```python
from build123d import *

# Parameters (mm, degrees)
CROQUIS1_R              = 2.55
CROQUIS1_R_2            = 1.55
SALIENTE_EXTRUIR1_DEPTH = 3
REDONDEO2_R             = 2
CORTAR_EXTRUIR1_DEPTH   = 3


with BuildPart() as part:
    # Croquis1 → Saliente-Extruir1 (new body)
    with BuildSketch(Plane(origin=(0, 0, 0), x_dir=(1, 0, 0), z_dir=(0, 1, 0))):
        Polygon((0, 0), (300, 0), (300, 30), (292, 30), (292, 38), (278, 38), (278, 30), (165, 30), (165, 35), (135, 35), (135, 30), (22, 30), (22, 38), (8, 38), (8, 30), (0, 30), align=None)
        with Locations((3.4, 26.6)):
            Circle(CROQUIS1_R, mode=Mode.SUBTRACT)
        with Locations((26.6, 26.6)):
            Circle(CROQUIS1_R, mode=Mode.SUBTRACT)
        with Locations((26.6, 3.4)):
            Circle(CROQUIS1_R, mode=Mode.SUBTRACT)
        with Locations((3.4, 3.4)):
            Circle(CROQUIS1_R, mode=Mode.SUBTRACT)
        with Locations((273.4, 3.4)):
            Circle(CROQUIS1_R, mode=Mode.SUBTRACT)
        with Locations((296.6, 3.4)):
            Circle(CROQUIS1_R, mode=Mode.SUBTRACT)
        with Locations((296.6, 26.6)):
            Circle(CROQUIS1_R, mode=Mode.SUBTRACT)
        with Locations((273.4, 26.6)):
            Circle(CROQUIS1_R, mode=Mode.SUBTRACT)
        with Locations((150, 30)):
            Circle(CROQUIS1_R_2, mode=Mode.SUBTRACT)
        with Locations((150, 10)):
            Circle(CROQUIS1_R_2, mode=Mode.SUBTRACT)
        with Locations((120, 23)):
            Circle(CROQUIS1_R_2, mode=Mode.SUBTRACT)
        with Locations((120, 8)):
            Circle(CROQUIS1_R_2, mode=Mode.SUBTRACT)
        with Locations((180, 8)):
            Circle(CROQUIS1_R_2, mode=Mode.SUBTRACT)
        with Locations((180, 23)):
            Circle(CROQUIS1_R_2, mode=Mode.SUBTRACT)
    extrude(amount=SALIENTE_EXTRUIR1_DEPTH)

    # Redondeo2
    redondeo2_edges = [part.edges().sort_by_distance(p)[0] for p in [
        (0, 1.5, -30),
        (8, 1.5, -30),
        (8, 1.5, -38),
        (22, 1.5, -38),
        (22, 1.5, -30),
        (135, 1.5, -30),
        (135, 1.5, -35),
        (165, 1.5, -35),
        (165, 1.5, -30),
        (278, 1.5, -30),
        (278, 1.5, -38),
        (292, 1.5, -38),
        (292, 1.5, -30),
        (300, 1.5, -30),
        (300, 1.5, 0),
        (0, 1.5, 0),
    ]]
    fillet(redondeo2_edges, radius=REDONDEO2_R)

    # Croquis2 → Cortar-Extruir1 (cut)
    with BuildSketch(Plane(origin=(0, 3, 0), x_dir=(1, 0, 0), z_dir=(0, 1, 0))):
        with BuildLine():
            Line((135, 0), (165, 0))
            Line((165, 0), (165, 1.5))
            ThreePointArc((165, 1.5), (164.707106781, 2.207106781), (164, 2.5))
            Line((164, 2.5), (136, 2.5))
            ThreePointArc((136, 2.5), (135.292893219, 2.207106781), (135, 1.5))
            Line((135, 1.5), (135, 0))
        make_face()
    extrude(amount=-CORTAR_EXTRUIR1_DEPTH, mode=Mode.SUBTRACT)


solid = part.part
```
Geometry: final body of the model. Coordinates: model frame, mm. Coordinates: 2 decimals unless noted, no trailing zeros. Order: outer loops, then holes, each group sorted by start corner. A loop starts at its lowest first (then second) coordinate and runs counter-clockwise, first axis right, second up.
Item 1: Draft query along Z for faces 1 (the face through (148, 3, -15)), 2 (the face through (299.03, 1.48, -4.17)). Return one class per face: released by +Z, released by -Z, zero draft, split by the parting line, or undercut.
Answer:
face 1: zero draft
face 2: undercut
Item 2: Section query B-B (x = 100). Output: boundary loops of the cut face in (y, z), then the cut area to 3 significant figures.
Answer:
outline: (0, -30) - (3, -30) - (3, 0) - (0, 0) - close
area: 90.0 mm2
Item 3: Section query A-A (y = 1.65). State how many separate pieces and enclosed holes the cut face has, then the cut area to 3 significant figures.
Answer:
separate pieces: 1
enclosed holes: 14
area: 9,090 mm2
Item 4: Contact query for flat-ended pins moving along their axis: P1, Ø1.9, axis at x = 180, z = -23, coming from the +Y side; P2, Ø1, axis at x = 112, y = 2, coming from the -Z side; P3, Ø1.5, axis at y = 0.5, z = -30, coming from the -X side. Output: stop coordinate, or through.
Answer:
P1: passes through
P2: stops at z = -30
P3: stops at x = 0.44
Item 5: Material intervals for line 1 along Z through (x, y) = (180, 0.6); line 2 along X through (y, z) = (1.45, -26.6); line 3 along Z through (x, y) = (26.6, 1.5), sorted ascending.
Answer:
line 1: z = -30 to -24.55, -21.45 to -9.55, -6.45 to 0
line 2: x = 0 to 0.85, 5.95 to 24.05, 29.15 to 270.85, 275.95 to 294.05, 299.15 to 300
line 3: z = -30 to -29.15, -24.05 to -5.95, -0.85 to 0
